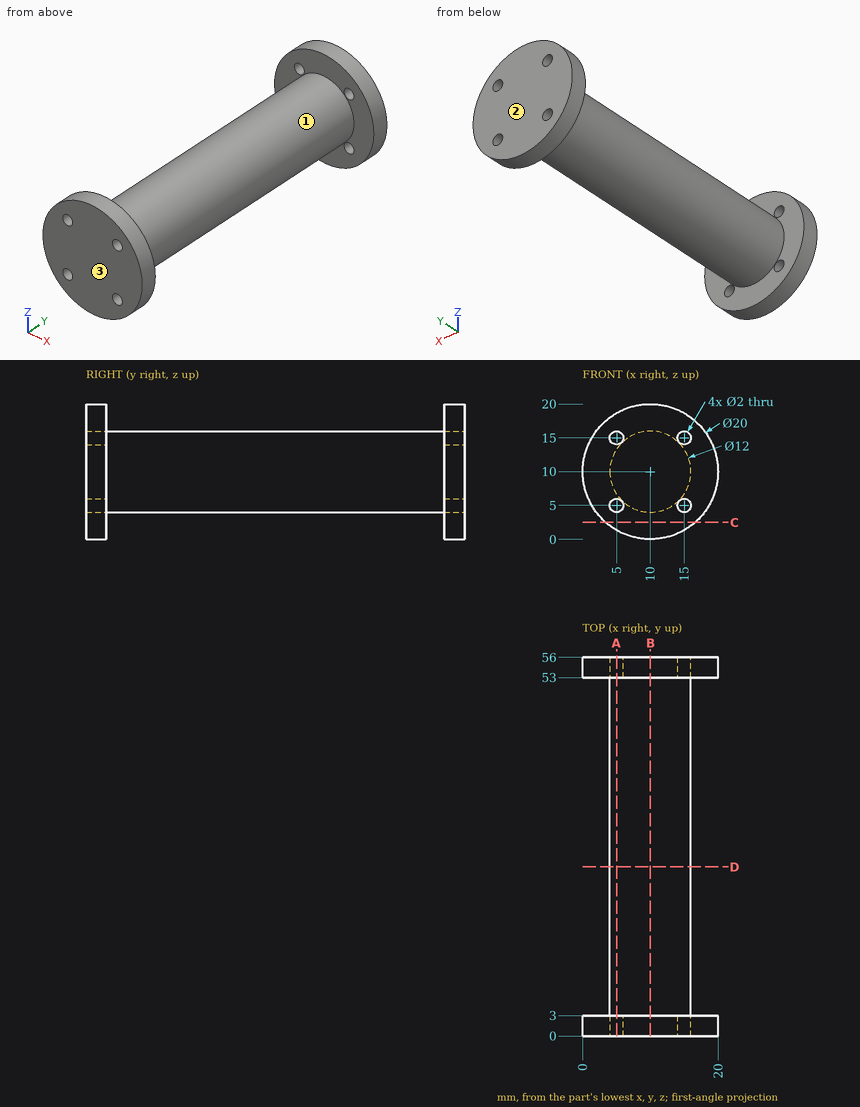
Geometry: see drawing. Coordinates: mm, zero at the bounding-box minimum. Coordinates: 2 decimals unless noted, no trailing zeros. Loops run counter-clockwise (first coordinate to the right, second up) from the corner with the lowest first, then second, coordinate; pieces in that order, holes last. Notation, with made-up numbers: M 45.25,17.25 L 74.25,17.25 A12 cw 74.25,23.25 Z; hole C 36.5,61 d5. An arc over 180 degrees is marked long. Answer in a Markdown table with one row per item.
Q1. Section C-C on z = 2.5. Return the cut outline in (x, y).
Answers below:
| item | result |
|---|---|
| outline | M 3.39,0 L 16.61,0 L 16.61,3 L 3.39,3 Z; M 3.39,53 L 16.61,53 L 16.61,56 L 3.39,56 Z |
Q2. Ray query, probe 1 along Y at (x, z) = (2.75, 13.5); probe 2 along Z at (x, y) = (5, 54.45); probe 3 along Z at (x, y) = (4.25, 53.5). Return the intervals inside material, ascending. Write a range as from..to.
Answers below:
| item | result |
|---|---|
| probe 1 | y = 0..3, 53..56 |
| probe 2 | z = 1.34..4, 6..14, 16..18.66 |
| probe 3 | z = 1.82..4.34, 5.66..14.34, 15.66..18.18 |
Q3. Draft query along Y for the marked faces 1, 2 and 3. Return one class per face: pulls with the +Y half, pulls with the -Y half, needs draft (parallel to the pull), parting line crosses it, or undercut.
Answers below:
| item | result |
|---|---|
| face 1 | undercut |
| face 2 | pulls with the +Y half |
| face 3 | pulls with the -Y half |
Q4. Section D-D on y = 25. Return the cut outline in (x, z), plus the area to 3 significant figures.
Answers below:
| item | result |
|---|---|
| outline | C 10,10 d12 |
| area | 113 mm^2 |
Q5. Section A-A on x = 5. Return the cut outline in (y, z).
Answers below:
| item | result |
|---|---|
| outline | M 0,1.34 L 3,1.34 L 3,4 L 0,4 Z; M 0,6 L 3,6 L 3,6.68 L 53,6.68 L 53,6 L 56,6 L 56,14 L 53,14 L 53,13.32 L 3,13.32 L 3,14 L 0,14 Z; M 0,16 L 3,16 L 3,18.66 L 0,18.66 Z; M 53,1.34 L 56,1.34 L 56,4 L 53,4 Z; M 53,16 L 56,16 L 56,18.66 L 53,18.66 Z |
Q6. Section B-B on x = 10. Return the cut outline in (y, z).
Answers below:
| item | result |
|---|---|
| outline | M 0,0 L 3,0 L 3,4 L 53,4 L 53,0 L 56,0 L 56,20 L 53,20 L 53,16 L 3,16 L 3,20 L 0,20 Z |
Q7. First-contact query: pin 1 (12 mm diameter, centred on y = 46, z = 13, fed in from +X); pin 2 (10 mm diameter, centred on x = 15, y = 27.5, fed in from +Z); pin 3 (5 mm diameter, centred on x = 2.5, y = 23, fed in from -Z). Flat tips, straight axial feed; report the tip coordinate or a pass-through.
Answers below:
| item | result |
|---|---|
| pin 1 | stops at x = 16 |
| pin 2 | stops at z = 16 |
| pin 3 | stops at z = 6.68 |
